```python
from build123d import *

# Parameters (mm, degrees)
SKETCH2_R               = 4.1
BOSS_EXTRUDE1_DEPTH     = 3.9
CUT_EXTRUDE1_DEPTH      = 7.987846592
BOSS_EXTRUDE2_DEPTH     = 7.5
CUT_EXTRUDE2_DEPTH      = 15.263590011
CUT_EXTRUDE2_DEPTH_BACK = 15.263590011
SKETCH5_R               = 1.075
CUT_EXTRUDE3_DEPTH      = 15.263590166
BOSS_EXTRUDE3_DEPTH     = 1.05
CUT_EXTRUDE4_DEPTH      = 13.370125448
CUT_EXTRUDE5_REACH      = 14.624
SKETCH9_R               = 0.85


with BuildPart() as part:
    # Sketch2 → Boss-Extrude1 (new body)
    with BuildSketch(Plane(origin=(0, 0, 0), x_dir=(1, 0, 0), z_dir=(0, 1, 0))):
        with Locations(Location((0, 0, 0), (0, 0, 270))):
            Circle(SKETCH2_R)
    extrude(amount=BOSS_EXTRUDE1_DEPTH)

    # Sketch3 → Cut-Extrude1 (cut, through all)
    with BuildSketch(Plane(origin=(0, 3.9, 0), x_dir=(1, 0, 0), z_dir=(0, 1, 0))):
        with BuildLine():
            Line((-2.5, 3.249615362), (-2.5, -3.249615362))
            ThreePointArc((-2.5, -3.249615362), (-4.1, 0), (-2.5, 3.249615362))
        make_face()
        with BuildLine():
            Line((2.5, 3.249615362), (2.5, -3.249615362))
            ThreePointArc((2.5, -3.249615362), (4.1, 0), (2.5, 3.249615362))
        make_face()
    extrude(amount=-CUT_EXTRUDE1_DEPTH, mode=Mode.SUBTRACT)

    # Sketch4 → Boss-Extrude2 (add)
    with BuildSketch(Plane(origin=(0, 3.9, 0), x_dir=(1, 0, 0), z_dir=(0, 1, 0))):
        with BuildLine():
            Line((-2.5, -3.249615362), (2.5, -3.249615362))
            ThreePointArc((2.5, -3.249615362), (0, -4.1), (-2.5, -3.249615362))
        make_face()
        with BuildLine():
            Line((-2.5, 3.249615362), (2.5, 3.249615362))
            ThreePointArc((2.5, 3.249615362), (0, 4.1), (-2.5, 3.249615362))
        make_face()
    extrude(amount=BOSS_EXTRUDE2_DEPTH)

    # Sketch5 → Cut-Extrude2 (cut, two sides: drawn at the far end of the back side and taken through both)
    with BuildSketch(Plane.XY.offset(4.1).offset(-CUT_EXTRUDE2_DEPTH_BACK)):
        with Locations(Location((0, 8.075, 0), (0, 0, 270))):
            Circle(SKETCH5_R)
    extrude(amount=CUT_EXTRUDE2_DEPTH + CUT_EXTRUDE2_DEPTH_BACK, mode=Mode.SUBTRACT)

    # Sketch6 → Cut-Extrude3 (cut, through all)
    with BuildSketch(Plane.XY.offset(4.1)):
        with BuildLine():
            Line((-2.5, 9.9), (-2.5, 11.4))
            Line((-2.5, 11.4), (0, 11.4))
            ThreePointArc((0, 11.4), (-1.457737974, 10.996229956), (-2.5, 9.9))
        make_face()
    cut_extrude3 = extrude(amount=-CUT_EXTRUDE3_DEPTH, mode=Mode.SUBTRACT)

    # Mirror1: Cut-Extrude3 across plane
    add(cut_extrude3.mirror(Plane(origin=(0, 0, 0), x_dir=(0, 0, 1), z_dir=(1, 0, 0))), mode=Mode.SUBTRACT)

    # Sketch7 → Boss-Extrude3 (add, symmetric)
    with BuildSketch(Plane(origin=(0, 0, 0), x_dir=(0, 0, -1), z_dir=(1, 0, 0))):
        with BuildLine():
            Line((4.1, 0), (-4.1, 0))
            ThreePointArc((-4.1, 0), (-3.845898176, -1.328520002), (-3.11946367, -2.469495917))
            ThreePointArc((-3.11946367, -2.469495917), (-2.754870811, -2.951250255), (-2.502108249, -3.5))
            ThreePointArc((-2.502108249, -3.5), (0, -5.3), (2.502108249, -3.5))
            ThreePointArc((2.502108249, -3.5), (2.754870811, -2.951250255), (3.11946367, -2.469495917))
            ThreePointArc((3.11946367, -2.469495917), (3.845898176, -1.328520002), (4.1, 0))
        make_face()
    extrude(amount=BOSS_EXTRUDE3_DEPTH, both=True)

    # Sketch8 → Cut-Extrude4 (cut, through all)
    with BuildSketch(Plane(origin=(0, 0, 0), x_dir=(1, 0, 0), z_dir=(0, 1, 0))):
        with BuildLine():
            Line((-1.05, -3.963268853), (-1.05, -4.1))
            Line((-1.05, -4.1), (0, -4.1))
            ThreePointArc((0, -4.1), (-0.529432575, -4.065673517), (-1.05, -3.963268853))
        make_face()
        with BuildLine():
            Line((-1.05, 4.1), (0, 4.1))
            ThreePointArc((0, 4.1), (-0.529432575, 4.065673517), (-1.05, 3.963268853))
            Line((-1.05, 3.963268853), (-1.05, 4.1))
        make_face()
    cut_extrude4 = extrude(amount=-CUT_EXTRUDE4_DEPTH, mode=Mode.SUBTRACT)

    # Mirror2: Cut-Extrude4 across plane
    add(cut_extrude4.mirror(Plane(origin=(0, 0, 0), x_dir=(0, 0, 1), z_dir=(1, 0, 0))), mode=Mode.SUBTRACT)

    # Sketch9 → Cut-Extrude5 (cut, up to next)
    with BuildSketch(Plane(origin=(1.05, 0, 0), x_dir=(0, 0, -1), z_dir=(1, 0, 0)), mode=Mode.PRIVATE) as cut_extrude5_sk1:
        with Locations((0, -2.7)):
            Circle(SKETCH9_R)
    cut_extrude5_tool1 = extrude(cut_extrude5_sk1.sketch, amount=-CUT_EXTRUDE5_REACH, mode=Mode.PRIVATE) & part.part
    add(cut_extrude5_tool1.solids().sort_by_distance((1.05, -2.7, 0))[0], mode=Mode.SUBTRACT)


solid = part.part
```
Check sheet for the modelled part. Datum: model origin and axes. Units: mm. A direction names the side the tool comes from. Round coordinates to 2 decimals unless told otherwise and drop trailing zeros. Write each loop counter-clockwise with the first axis right and the second up, starting at its lowest first coordinate (ties: lowest second). Pieces come first, ordered by that corner, then holes. Notation, with made-up numbers: (-33, 62.5) -> (24, 62.5) arc R24 ccw to (24, 93.5) -> close; hole circle Ø10 at (-7, 48.5). An arc over 180 degrees is marked (long way). Put each result on its own line as item: value.
(1) Sectioned sample at D-D (y = 7.75). Enter the section's corners in (x, z).
Values found:
outline: (-2.5, -3.25) arc R4.1 ccw to (-1.02, -3.97) -> (-1.02, -3.25) -> close; (-2.5, 3.25) -> (-1.02, 3.25) -> (-1.02, 3.97) arc R4.1 ccw to start; (1.02, -3.97) arc R4.1 ccw to (2.5, -3.25) -> (1.02, -3.25) -> close; (1.02, 3.25) -> (2.5, 3.25) arc R4.1 ccw to (1.02, 3.97) -> close
(2) Sectioned sample at A-A (z = 0). Enter the section's corners in (x, y), plus the area to 3 significant figures.
Values found:
outline: (-2.5, 0) -> (-1.05, 0) -> (-1.05, -1.85) -> (1.05, -1.85) -> (1.05, 0) -> (2.5, 0) -> (2.5, 3.9) -> (-2.5, 3.9) -> close; (-1.05, -5.3) -> (1.05, -5.3) -> (1.05, -3.55) -> (-1.05, -3.55) -> close
area: 27.1 mm^2
(3) Mould release check, pull along Y, two halves, no side actions. Record for faces 1 (the face through (0.32, 7.05, -3.68)), 2 (the face through (-2.5, 2, 0)), 3 (the face through (0, -5.3, 0)): released by +Y, released by -Y, zero draft, split by the parting line, or undercut.
Values found:
face 1: undercut
face 2: zero draft
face 3: released by -Y
(4) Sectioned sample at B-B (y = -2.7). Enter the section's corners in (x, z).
Values found:
outline: (-1.05, -2.92) -> (1.05, -2.92) -> (1.05, -0.85) -> (-1.05, -0.85) -> close; (-1.05, 0.85) -> (1.05, 0.85) -> (1.05, 2.92) -> (-1.05, 2.92) -> close
(5) Tool access check on faces 4 (the face through (-1.05, -1, 0)), 5 (the face through (0.32, 7.05, 3.67)), 6 (the face through (0.01, -2.94, 2.76)), 7 (the face through (1.05, -1, 0)), 8 (the face through (0, 6.8, -3.25)). Record the directions out of +Z, -Z, +X, -X, +Y, -Y that give a thin tool (end or side, any length) a straight path to the whole face; none if there is none.
Values found:
face 4: +Z, -Z, -X, -Y
face 5: +Z, -Z
face 6: +Z, +X, -X, -Y
face 7: +Z, -Z, +X, -Y
face 8: +X, -X, +Y
(6) Sectioned sample at C-C (x = 1.4). Enter the section's corners in (y, z), plus the area to 3 significant figures.
Values found:
outline: (0, -3.85) -> (11.03, -3.85) -> (11.03, -3.25) -> (3.9, -3.25) -> (3.9, 3.25) -> (11.03, 3.25) -> (11.03, 3.85) -> (0, 3.85) -> close
area: 38.7 mm^2
(7) Go/stop test with flat-tipped pins: pin 1 Ø2 at (x, y) = (-1.5, -3) entering from +Z; pin 2 Ø2.5 at (y, z) = (-3, 0.5) entering from -X; pin 3 Ø2 at (x, y) = (-0.5, 8) entering from +Z. Record where each tip stops, or that it passes through.
Values found:
pin 1: stops at z = 3.42
pin 2: stops at x = -1.05
pin 3: stops at z = 4.09
(8) Material ranges on line 1 (Y direction, x = -1.2, z = 0.25); line 2 (Y direction, x = 0, z = -3.7); line 3 (Z direction, x = 0.15, y = -2.75), recorded low to high.
Values found:
line 1: y = 0 to 3.9
line 2: y = -1.65 to 7, 9.15 to 11.4
line 3: z = -2.89 to -0.85, 0.85 to 2.89
